from build123d import *

# Parameters (mm, degrees)
SKETCH1_W           = 38.1
SKETCH1_H           = 12.7
SKETCH1_R           = 1.190625
BOSS_EXTRUDE1_DEPTH = 3.175
SKETCH2_W           = 38.1
SKETCH2_H           = 15.875
BOSS_EXTRUDE2_DEPTH = 3.175
FILLET1_R           = 3.175
FILLET2_R           = 0.381
SKETCH3_R           = 1.190625
CUT_EXTRUDE1_DEPTH  = 16.557632845
SKETCH4_R           = 1.190625
CUT_EXTRUDE2_DEPTH  = 13.7


with BuildPart() as part:
    # Sketch1 → Boss-Extrude1 (new body)
    with BuildSketch(Plane.XY):
        with Locations((19.05, -6.35)):
            Rectangle(SKETCH1_W, SKETCH1_H)
        with Locations((9.525, -3.175)):
            Circle(SKETCH1_R, mode=Mode.SUBTRACT)
        with Locations((28.575, -3.175)):
            Circle(SKETCH1_R, mode=Mode.SUBTRACT)
    extrude(amount=BOSS_EXTRUDE1_DEPTH)

    # Sketch2 → Boss-Extrude2 (add)
    with BuildSketch(Plane(origin=(0, -12.7, 0), x_dir=(-1, 0, 0), z_dir=(0, -1, 0))):
        with Locations((-19.05, -11.1125)):
            Rectangle(SKETCH2_W, SKETCH2_H)
    extrude(amount=-BOSS_EXTRUDE2_DEPTH)

    # Fillet1
    fillet1_edges = [part.edges().sort_by_distance(p)[0] for p in [
        (38.1, 0, 1.5875),
        (0, 0, 1.5875),
        (19.05, -9.525, 3.175),
        (38.1, -11.1125, 19.05),
        (0, -11.1125, 19.05),
    ]]
    fillet(fillet1_edges, radius=FILLET1_R)

    # Fillet2
    fillet2_edges = [part.edges().sort_by_distance(p)[0] for p in [
        (19.05, 0, 3.175),
        (38.1, -4.7625, 3.175),
        (38.1, -9.525, 11.1125),
        (0, -4.7625, 3.175),
        (0.92993597, -0.92993597, 3.175),
        (37.17006403, -0.92993597, 3.175),
        (0, -9.525, 11.1125),
        (19.05, -9.525, 19.05),
        (0.92993597, -9.525, 18.12006403),
        (37.17006403, -9.525, 18.12006403),
        (38.1, -8.59506403, 4.10493597),
        (0, -8.59506403, 4.10493597),
    ]]
    fillet(fillet2_edges, radius=FILLET2_R)

    # Sketch3 → Cut-Extrude1 (cut, through all)
    with BuildSketch(Plane(origin=(0, 4.650907684, 4.650907684), x_dir=(-1, 0, 0), z_dir=(0, 0.707106781, 0.707106781))):
        with Locations((-19.05, 16.664983956)):
            Circle(SKETCH3_R)
    extrude(amount=-CUT_EXTRUDE1_DEPTH, mode=Mode.SUBTRACT)

    # Sketch4 → Cut-Extrude2 (cut, through all)
    with BuildSketch(Plane(origin=(0, -12.7, 0), x_dir=(-1, 0, 0), z_dir=(0, -1, 0))):
        with Locations((-9.525, -12.7)):
            Circle(SKETCH4_R)
        with Locations((-28.575, -12.7)):
            Circle(SKETCH4_R)
    extrude(amount=-CUT_EXTRUDE2_DEPTH, mode=Mode.SUBTRACT)


solid = part.part
For this review, take the finished solid that the model builds, in its own axes (mm). A direction names the side the tool comes from. Round coordinates to 2 decimals unless told otherwise and drop trailing zeros. Loops run counter-clockwise (first coordinate to the right, second up) from the corner with the lowest first, then second, coordinate; pieces in that order, holes last. Notation, with made-up numbers: (3, -23) - (27, -23) arc R27 cw to (27, 15) - close; hole circle Ø10 at (59.5, 36). An arc over 180 degrees is marked (long way). Put each result on its own line as item: value. Start each with the question number.
1. Consider section C-C on z = 7. State the section outline as (x, y) points (3 decimals).
2. For faces 5 (the cylindrical face through (37.19, -0.95, 1.42)), 6 (the flat face through (19, -9.525, 11)), list the 3-axis set-ups (+Z, -Z, +X, -X, +Y, -Y) from which the entire face can be reached by the end or side of a thin tool; tool diameter is ignored.
3. Consider section A-A on z = 2. State the section outline as (x, y) points (3 decimals).
4. Mouldability with a two-part tool opening along Y and no side actions: class faces 1 (the cylindrical face through (18.79, -8.57, 4.08)), 2 (the cylindrical face through (29.71, -2.82, 1.57)), 3 (the flat face through (19, -11, 19.05)), 4 (the cylindrical face through (10.66, -2.82, 1.57)) as +Y half, -Y half, draft (parallel to the pull), parting line (faces both ways), or undercut.
5. For probe 1 along X at (y, z) = (-11.1, 12.7); probe 2 along Y at (x, z) = (11, 11) (3 decimals); probe 3 along Z at (x, y) = (24.5, -3.25) (3 decimals), list the stretches that pass through material, from the lowest coordinate up. Write a range as [from, to].
6. Consider section B-B on x = 19. State the section outline as (y, z) points (3 decimals).
7. Insertion check: P1, Ø5, axis at x = 12, z = 12.5, coming from the +Y side (3 decimals); P2, Ø3, axis at x = 9.525, y = -3.175, coming from the +Z side (3 decimals). Each pin has a flat end and moves straight along its axis. Give the tip position at first contact, or say it passes through.
Result sheet:
1. outline: (0, -12.7) - (38.1, -12.7) - (38.1, -9.906) arc R0.381 ccw to (37.719, -9.525) - (0.381, -9.525) arc R0.381 ccw to (0, -9.906) - close
2. face 5: +Z, -Z, +X, +Y
2. face 6: +Z, +X, -X, +Y
3. outline: (0, -12.7) - (38.1, -12.7) - (38.1, -3.175) arc R3.175 ccw to (34.925, 0) - (3.175, 0) arc R3.175 ccw to (0, -3.175) - close; hole circle Ø2.381 at (9.525, -3.175); hole circle Ø2.381 at (28.575, -3.175)
4. face 1: +Y half
4. face 2: undercut
4. face 3: draft
4. face 4: undercut
5. probe 1: [0, 8.33], [10.72, 17.87], [20.23, 27.38], [29.77, 38.1]
5. probe 2: [-12.7, -9.525]
5. probe 3: [0, 3.175]
6. outline: (-12.7, 0) - (0, 0) - (0, 2.794) arc R0.381 ccw to (-0.381, 3.175) - (-6.35, 3.175) arc R3.175 cw to (-9.525, 6.35) - (-9.525, 12.361) - (-12.7, 9.186) - close; (-12.7, 12.55) - (-9.525, 15.725) - (-9.525, 18.669) arc R0.381 ccw to (-9.906, 19.05) - (-12.7, 19.05) - close
7. P1: y = -9.525
7. P2: z = 3.175
